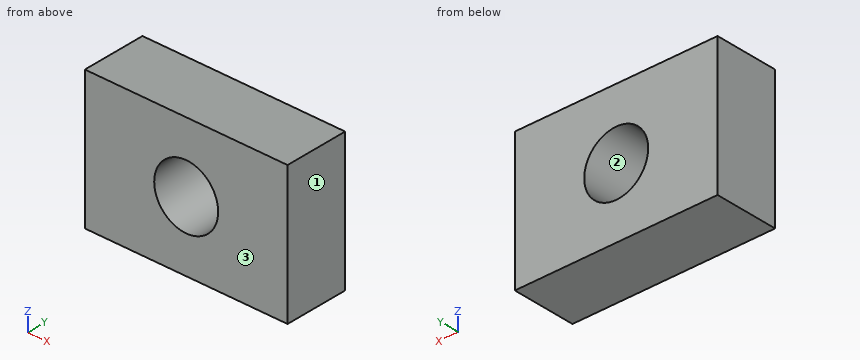
Autodesk Inventor part; units mm, degrees
ref_plane "YZ Plane" through (0, 0, 0) normal (1, 0, 0) x (0, 1, 0)
ref_plane "XZ Plane" through (0, 0, 0) normal (0, 1, 0) x (-1, 0, 0)
ref_plane "XY Plane" through (0, 0, 0) normal (0, 0, 1) x (1, 0, 0)
sketch "Sketch1" plane through (0, 0, 0) normal (0, 1, 0) x (-1, 0, 0)
  line L0 (4.75, 3.25) -> (-4.75, 3.25)
  line L1 (-4.75, 3.25) -> (-4.75, -3.25)
  line L2 (-4.75, -3.25) -> (4.75, -3.25)
  line L3 (4.75, -3.25) -> (4.75, 3.25)
  line L4 (4.75, 3.25) -> (-4.75, -3.25) construction
  line L5 (-4.75, 3.25) -> (4.75, -3.25) construction
  circle A0 centre (0, 0) radius 1.5
  dimension "d0" = 9.5
  dimension "d1" = 6.5
  dimension "d2" = 3
extrude "Extrusion1" add sketch "Sketch1" along normal blind 3
thread "Thread1"
properties material "Brass, Soft Yellow, Welded"
Could you check a few things on this model? Use its own coordinates, in mm. Face numbers are marked on the shaded views. Give positions to 0.01 mm unless a question says otherwise; leave off trailing zeros. Order: outer loops, then holes, each group sorted by start corner. A loop starts at its lowest first (then second) coordinate and runs counter-clockwise, first axis right, second up. Notation, with made-up numbers: (44, 16) - (69, 16) arc R16 ccw to (69, 47) - close; hole circle Ø9 at (62, 17.5). An arc over 180 degrees is marked (long way). Return JSON: item names as keys, results as strings. Group by question number.
Q1. Suppose I cut it at C-C, the plane y = 1.4. Please give me the cut outline in (x, z), and give its area (3 significant figures).
Q2. Suppose I cut it at B-B, the plane x = 0. Please give me the cut outline in (y, z).
Q3. Suppose I cut it at A-A, the plane z = 0. Please give me the cut outline in (x, y), and give its area (3 significant figures).
Q4. Please list where these lines run through material, in increasing order: line 1 along Z through (x, y) = (0, 1.8); line 2 along Z through (x, y) = (0.5, 1.85); line 3 along X through (y, z) = (1.1, 1.25). Write a range as [from, to].
Q5. Thinking about a two-plate mould opening in X: for the marked faces 1, 2 and 3, which applies, pulls with the +X half, pulls with the -X half, needs draft (parallel to the pull), parting line crosses it, or undercut?
Resolved:
{
 "1": {"outline": "(-4.75, -3.25) - (4.75, -3.25) - (4.75, 3.25) - (-4.75, 3.25) - close; hole circle Ø3 at (0, 0)", "area": "54.7 mm2"},
 "2": {"outline": "(0, -3.25) - (3, -3.25) - (3, -1.5) - (0, -1.5) - close; (0, 1.5) - (3, 1.5) - (3, 3.25) - (0, 3.25) - close"},
 "3": {"outline": "(-4.75, 0) - (-1.5, 0) - (-1.5, 3) - (-4.75, 3) - close; (1.5, 0) - (4.75, 0) - (4.75, 3) - (1.5, 3) - close", "area": "19.5 mm2"},
 "4": {"line 1": "z = [-3.25, -1.5], [1.5, 3.25]", "line 2": "z = [-3.25, -1.41], [1.41, 3.25]", "line 3": "x = [-4.75, -0.83], [0.83, 4.75]"},
 "5": {"face 1": "pulls with the +X half", "face 2": "undercut", "face 3": "needs draft"}
}
